Geometry check sheet. Reference: the model listing, model coordinates, mm. Face numbers are marked on the shaded views. A direction names the side the tool comes from. Give positions to 0.01 mm unless a question says otherwise; leave off trailing zeros. Write each loop counter-clockwise with the first axis right and the second up, starting at its lowest first coordinate (ties: lowest second). Pieces come first, ordered by that corner, then holes.
(1) Cross-section at C-C (x = -33.5). Record the boundary of the cut face in (y, z).
(2) Cross-section at B-B (y = -15.5). Record the boundary of the cut face in (x, z).
(3) Cross-section at A-A (z = 0). Record the boundary of the cut face in (x, y), and give its area (3 significant figures).
(4) Tool access check on the marked faces 1, 2, 3 and 4. Record the directions out of +Z, -Z, +X, -X, +Y, -Y that give a thin tool (end or side, any length) a straight path to the whole face; none if there is none.
(5) Thickness scan on line 1 along Z through (x, y) = (20, -13.5); line 2 along Y through (x, z) = (5, 26); line 3 along Z through (x, y) = (-8, 32). Record the ranges inside material, lowest first.
(6) Depth check by flat-ended pin: P1, Ø2, axis at x = -8.5, z = 27.5, coming from the -Y side; P2, Ø3, axis at x = -34, z = -16.5, coming from the +Y side; P3, Ø5, axis at x = 19.5, y = -46.5, coming from the -Z side. Enter the tip coordinate at first touch or a pass-through.
(7) Cross-section at D-D (x = 0). Record the boundary of the cut face in (y, z).
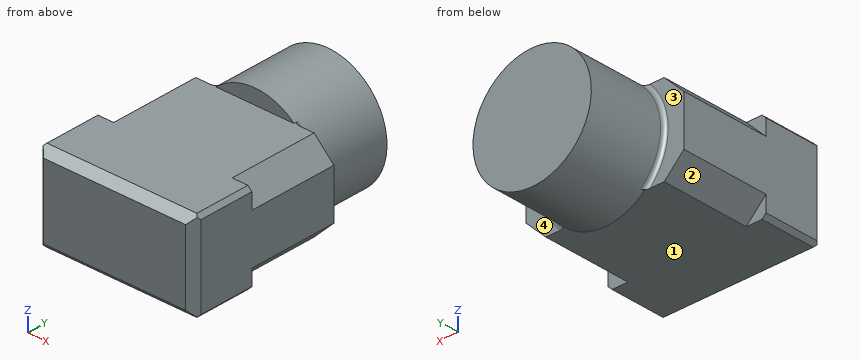
```python
from build123d import *

# Parameters (mm, degrees)
SKETCH1_R           = 30
BOSS_EXTRUDE1_DEPTH = 40
SKETCH2_W           = 80
SKETCH2_H           = 45
BOSS_EXTRUDE2_DEPTH = 45
CHAMFER1_SIZE       = 10
SKETCH4_W           = 80
SKETCH4_H           = 45
BOSS_EXTRUDE3_DEPTH = 2
SKETCH5_W           = 80
SKETCH5_H           = 45
BOSS_EXTRUDE4_DEPTH = 30
CHAMFER2_SIZE       = 2
CHAMFER3_SIZE       = 4
FILLET1_R           = 2


with BuildPart() as part:
    # Sketch1 → Boss-Extrude1 (new body)
    with BuildSketch(Plane(origin=(0, 0, 0), x_dir=(1, 0, 0), z_dir=(0, 1, 0))):
        with Locations(Location((0, 0, 0), (0, 0, 270))):
            Circle(SKETCH1_R)
    extrude(amount=BOSS_EXTRUDE1_DEPTH)

    # Sketch2 → Boss-Extrude2 (add)
    with BuildSketch(Plane.XZ):
        Rectangle(SKETCH2_W, SKETCH2_H)
    extrude(amount=BOSS_EXTRUDE2_DEPTH)

    # Chamfer1
    chamfer1_edges = [part.edges().sort_by_distance(p)[0] for p in [
        (40, -22.5, 22.5),
        (-40, -22.5, 22.5),
        (-40, -22.5, -22.5),
        (40, -22.5, -22.5),
    ]]
    chamfer(chamfer1_edges, length=CHAMFER1_SIZE)

    # Sketch4 → Boss-Extrude3 (add)
    with BuildSketch(Plane(origin=(0, -45, 0), x_dir=(-1, 0, 0), z_dir=(0, -1, 0))):
        Rectangle(SKETCH4_W, SKETCH4_H)
    extrude(amount=BOSS_EXTRUDE3_DEPTH)

    # Sketch5 → Boss-Extrude4 (add)
    with BuildSketch(Plane.XZ.offset(47)):
        Rectangle(SKETCH5_W, SKETCH5_H)
    extrude(amount=BOSS_EXTRUDE4_DEPTH)

    # Chamfer2
    chamfer2_edges = [part.edges().sort_by_distance(p)[0] for p in [
        (40, -61, -22.5),
        (40, -61, 22.5),
        (-40, -61, 22.5),
        (-40, -61, -22.5),
    ]]
    chamfer(chamfer2_edges, length=CHAMFER2_SIZE)

    # Chamfer3
    # the kernel refuses this chamfer: 4 mm, written as the material it takes off along each edge
    with BuildSketch(Plane(origin=(48.286731952, -77, 22.5), x_dir=(0, 0.9996219169112968, 0.02749587661058651), z_dir=(-1, 0, 0))) as chamfer3_piece_1:
        Polygon((CHAMFER3_SIZE * 0.999621916911, CHAMFER3_SIZE * 0.0274958766106), (-CHAMFER3_SIZE * 0.0274958766106, CHAMFER3_SIZE * 0.999621916911), (0, 0), align=None)
    extrude(amount=96.573463904, mode=Mode.SUBTRACT)
    with BuildSketch(Plane(origin=(-40, -77, 30.786731952), x_dir=(0.9996219169112968, -0.027495876610585647, 0), z_dir=(0, 0, -1)), Plane(origin=(40, -77, -30.786731952), x_dir=(-0.9996219169112968, -0.027495876610585647, 0), z_dir=(0, 0, 1))) as chamfer3_piece_2:
        Polygon((CHAMFER3_SIZE * 0.999621916911, -CHAMFER3_SIZE * 0.0274958766106), (-CHAMFER3_SIZE * 0.0274958766106, -CHAMFER3_SIZE * 0.999621916911), (0, 0), align=None)
    extrude(amount=61.573463904, mode=Mode.SUBTRACT)
    with BuildSketch(Plane(origin=(-48.286731952, -77, -22.5), x_dir=(0, -0.027495876610585623, 0.9996219169112968), z_dir=(1, 0, 0))) as chamfer3_piece_3:
        Polygon((CHAMFER3_SIZE * 0.999621916911, -CHAMFER3_SIZE * 0.0274958766106), (-CHAMFER3_SIZE * 0.0274958766106, -CHAMFER3_SIZE * 0.999621916911), (0, 0), align=None)
    extrude(amount=96.573463904, mode=Mode.SUBTRACT)

    # Fillet1
    # the kernel refuses this fillet: 2 mm, written as the material it adds along each edge
    with BuildSketch(Plane(origin=(0, 0, 0), x_dir=(0.527784032478236, 0, 0.8493786052526943), z_dir=(-0.8493786052526943, 0, 0.527784032478236))) as fillet1_piece_1_section:
        with BuildLine():
            CenterArc((30 + FILLET1_R, FILLET1_R), FILLET1_R, 180, 90)
            Line((30, FILLET1_R), (30, 0))
            Line((30, 0), (30 + FILLET1_R, 0))
        make_face()
    fillet1_piece_1 = revolve(axis=Axis((0, 0, 0), (0, 1, 0)), revolution_arc=116.288294518, mode=Mode.PRIVATE)
    fillet1_piece_1 = split(fillet1_piece_1, bisect_by=Plane(origin=(30.560923214, 0.560923214, 22.5), z_dir=(0, 0, -1)), keep=Keep.TOP, mode=Mode.PRIVATE)
    fillet1_piece_1 = split(fillet1_piece_1, bisect_by=Plane(origin=(30.560923214, 0.560923214, -22.5), z_dir=(0, 0, 1)), keep=Keep.TOP, mode=Mode.PRIVATE)
    add(fillet1_piece_1)
    with BuildSketch(Plane(origin=(0, 0, 0), x_dir=(-0.527784032478229, 0, -0.8493786052526988), z_dir=(0.8493786052526988, 0, -0.527784032478229))) as fillet1_piece_2_section:
        with BuildLine():
            CenterArc((30 + FILLET1_R, FILLET1_R), FILLET1_R, 180, 90)
            Line((30, FILLET1_R), (30, 0))
            Line((30, 0), (30 + FILLET1_R, 0))
        make_face()
    fillet1_piece_2 = revolve(axis=Axis((0, 0, 0), (0, 1, 0)), revolution_arc=116.288294518, mode=Mode.PRIVATE)
    fillet1_piece_2 = split(fillet1_piece_2, bisect_by=Plane(origin=(-30.560923214, 0.560923214, 22.5), z_dir=(0, 0, -1)), keep=Keep.TOP, mode=Mode.PRIVATE)
    fillet1_piece_2 = split(fillet1_piece_2, bisect_by=Plane(origin=(-30.560923214, 0.560923214, -22.5), z_dir=(0, 0, 1)), keep=Keep.TOP, mode=Mode.PRIVATE)
    add(fillet1_piece_2)


solid = part.part
```
Reply:
1. outline: (-77, -18.5) - (-73, -22.5) - (-45, -22.5) - (-45, -19) - (0, -19) - (0, 19) - (-45, 19) - (-45, 22.5) - (-73, 22.5) - (-77, 18.5) - close
2. outline: (-40, -12.5) - (-30, -22.5) - (30, -22.5) - (40, -12.5) - (40, 12.5) - (30, 22.5) - (-30, 22.5) - (-40, 12.5) - close
3. outline: (-40, -73) - (-36, -77) - (36, -77) - (40, -73) - (40, 0) - (32, 0) arc R2 cw to (30, 2) - (30, 40) - (-30, 40) - (-30, 2) arc R2 cw to (-32, 0) - (-40, 0) - close
3. area: 8,550 mm2
4. face 1: -Z, +X, -X, -Y
4. face 2: -Z, -X, +Y
4. face 3: -X, +Y
4. face 4: +X, +Y
5. line 1: z = -22.5 to 22.5
5. line 2: y = 0 to 40
5. line 3: z = -28.91 to 28.91
6. P1: stops at y = 0
6. P2: stops at y = 0
6. P3: stops at z = -22.5
7. outline: (-77, -18.5) - (-73, -22.5) - (0, -22.5) - (0, -30) - (40, -30) - (40, 30) - (0, 30) - (0, 22.5) - (-73, 22.5) - (-77, 18.5) - close
